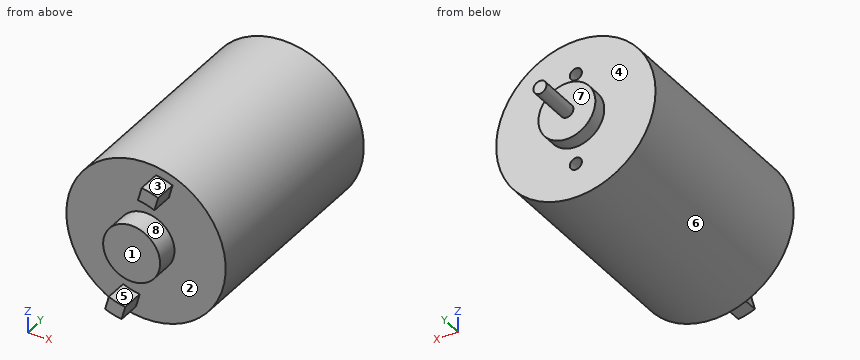
Autodesk Inventor part; units mm, degrees
ref_plane "YZ Plane" through (0, 0, 0) normal (1, 0, 0) x (0, 1, 0)
ref_plane "XZ Plane" through (0, 0, 0) normal (0, 1, 0) x (-1, 0, 0)
ref_plane "XY Plane" through (0, 0, 0) normal (0, 0, 1) x (1, 0, 0)
sketch "Sketch1" plane through (0, 0, 0) normal (0, 1, 0) x (-1, 0, 0)
  circle A0 centre (0, 0) radius 14
  dimension "d0" = 28
extrude "Extrusion1" add sketch "Sketch1" along normal blind 38.4
sketch "Sketch2" plane through (0, 38.4, 0) normal (0, 1, 0) x (1, 0, 0)
  circle A0 centre (0, 0) radius 5
  circle A1 centre (0, 0) radius 1.15
  circle A2 centre (0, 0) radius 8
  line L0 (0, -8) -> (0, 8)
  dimension "d3" = 10
  dimension "d6" = 2.3
  dimension "d9" = 16
extrude "Extrusion2" add sketch "Sketch2" along normal blind 2.5 contours A0 L0 A1 | L0 A1 A0 | L0 A1 | A1 L0
extrude "Extrusion3" add sketch "Sketch2" along normal blind 10 contours L0 A1 | A1 L0
hole "Hole1" at (0, 38.4, 8) at (0, 38.4, -8) direction (0, -1, 0) diameter 2.1129 depth 7.8
sketch "Sketch3" plane through (0, 0, 0) normal (0, -1, 0) x (1, 0, 0)
  circle A0 centre (0, 0) radius 5
  dimension "d17" = 10
extrude "Extrusion4" add sketch "Sketch3" along normal blind 4
sketch "Sketch4" plane through (0, 0, 0) normal (0, -1, 0) x (1, 0, 0)
  line L0 (-12.0122, 7.6623) -> (12.8258, 7.6623) construction
  line L1 (12.8258, 7.6623) -> (12.8258, -7.5309) construction
  line L2 (12.8258, -7.5309) -> (-12.0122, -7.5309) construction
  line L3 (-12.0122, -7.5309) -> (-12.0122, 7.6623) construction
  point P0 (0, 0)
sketch "Sketch5" plane through (0, 0, 0) normal (0, -1, 0) x (1, 0, 0)
  circle A0 centre (0, 8) radius 1.0564
  circle A1 centre (0, -8) radius 1.0564
  circle A2 centre (0, 0) radius 5
  circle A3 centre (0, 0) radius 14
  circle A4 centre (0, 0) radius 1.15
  circle A5 centre (0, 0) radius 12.5
  circle A6 centre (0, 0) radius 10
  line L0 (4.6607, 11.5986) -> (4.0078, 9.1617)
  line L1 (1.763, 12.3751) -> (1.11, 9.9382)
  line L2 (-1.11, -9.9382) -> (-1.763, -12.3751)
  line L3 (-4.0078, -9.1617) -> (-4.6607, -11.5986)
  line L4 (3.6235, 13.523) -> (-3.6235, -13.523)
  line L5 (0, 14) -> (0, -14) construction
  circle A7 centre (0, 0) radius 14
  dimension "d21" = 2.5
  dimension "d27" = 20
  dimension "d28" = 1.5
  dimension "d29" = 15
  dimension "d30" = 1.5
  dimension "d31" = 1.5
  dimension "d32" = 1.5
  dimension "d33" = 1.5
extrude "Extrusion5" add sketch "Sketch5" along normal up to surface (4 mm away) contours L4 A5 L0 A6 | A6 L1 A5 L4 | L4 A5 L3 A6 | A6 L2 A5 L4
equation "\"d31\" = d30"
equation "\"d32\" = d30"
properties part number "rs385"
Could you check a few things on this model? Use its own coordinates, in mm. Face numbers are marked on the shaded views. A direction names the side the tool comes from. Coordinates: 2 decimals unless noted, no trailing zeros. Loops run counter-clockwise (first coordinate to the right, second up) from the corner with the lowest first, then second, coordinate; pieces in that order, holes last. Notation, with made-up numbers: M -16,10.5 L -4,10.5 A30 cw -4,46.5 Z; hole C 82.25,29.5 d1. An arc over 180 degrees is marked long. Put each result on its own line as item: value. Start each with the question number.
(1) Will these pins go through, and if not, where does the flat tip stop? P1, Ø3, axis at x = -1, z = -2, coming from the +Y side; P2, Ø1.1, axis at x = 0.5, z = 7.5, coming from the +Y side; P3, Ø1.5, axis at x = -3, y = 37.5, coming from the -Z side; P4, Ø2.5, axis at x = 0, z = -8, coming from the -Y side.
(2) Thinking about a two-plate mould opening in Z: for the marked faces 6, 7 and 8, which applies, pulls with the +Z half, pulls with the -Z half, needs draft (parallel to the pull), parting line crosses it, or undercut?
(3) Suppose I cut it at D-D on z = 8. Please give me the cut outline in (x, y).
(4) I need wall thicknesses on line 1 (Z direction, x = 0, y = 33.75); line 2 (Y direction, x = -7.75, z = 6.25); line 3 (Z direction, x = -0.5, y = 22). Which ranges of each line are inside material? Lowest first, please. Write a range as from..to.
(5) Suppose I cut it at C-C on y = 19.5. Please give me the cut outline in (x, z), then the cut area to 3 significant figures.
(6) Suppose I cut it at A-A on z = 0. Please give me the cut outline in (x, y).
(7) For the marked faces 1, 2, 3, 4 and 5, which set-ups out of +Z, -Z, +X, -X, +Y, -Y let a thin tool reach every point of the face, with its end or its side?
(8) Suppose I cut it at B-B on x = 0. Please give me the cut outline in (y, z), then the cut area to 3 significant figures.
Solutions:
1. P1: stops at y = 48.4
1. P2: stops at y = 38.4
1. P3: stops at z = -13.82
1. P4: stops at y = 0
2. face 6: parting line crosses it
2. face 7: needs draft
2. face 8: undercut
3. outline: M -11.49,0 L 11.49,0 L 11.49,38.4 L 1.06,38.4 L 1.06,30.6 L -1.06,30.6 L -1.06,38.4 L -11.49,38.4 Z
4. line 1: z = -14..-9.06, -6.94..6.94, 9.06..14
4. line 2: y = 0..38.4
4. line 3: z = -13.99..13.99
5. outline: C 0,0 d28
5. area: 616 mm2
6. outline: M -14,0 L -5,0 L -5,-4 L 5,-4 L 5,0 L 14,0 L 14,38.4 L 5,38.4 L 5,40.9 L 1.15,40.9 L 1.15,48.4 L -1.15,48.4 L -1.15,40.9 L -5,40.9 L -5,38.4 L -14,38.4 Z
7. face 1: +Z, -Z, +X, -X, -Y
7. face 2: -Y
7. face 3: +Z, +X, -Y
7. face 4: +Y
7. face 5: +X, -Y
8. outline: M -4,-5 L 0,-5 L 0,-14 L 38.4,-14 L 38.4,-9.06 L 30.6,-9.06 L 30.6,-6.94 L 38.4,-6.94 L 38.4,-5 L 40.9,-5 L 40.9,-1.15 L 48.4,-1.15 L 48.4,1.15 L 40.9,1.15 L 40.9,5 L 38.4,5 L 38.4,6.94 L 30.6,6.94 L 30.6,9.06 L 38.4,9.06 L 38.4,14 L 0,14 L 0,5 L -4,5 Z
8. area: 1,120 mm2
